For this review, use the dimensioned drawing (mm, ordinates from the lowest corner) and the shaded views. Round coordinates to 2 decimals unless told otherwise and drop trailing zeros. Write each loop counter-clockwise with the first axis right and the second up, starting at its lowest first coordinate (ties: lowest second). Pieces come first, ordered by that corner, then holes.
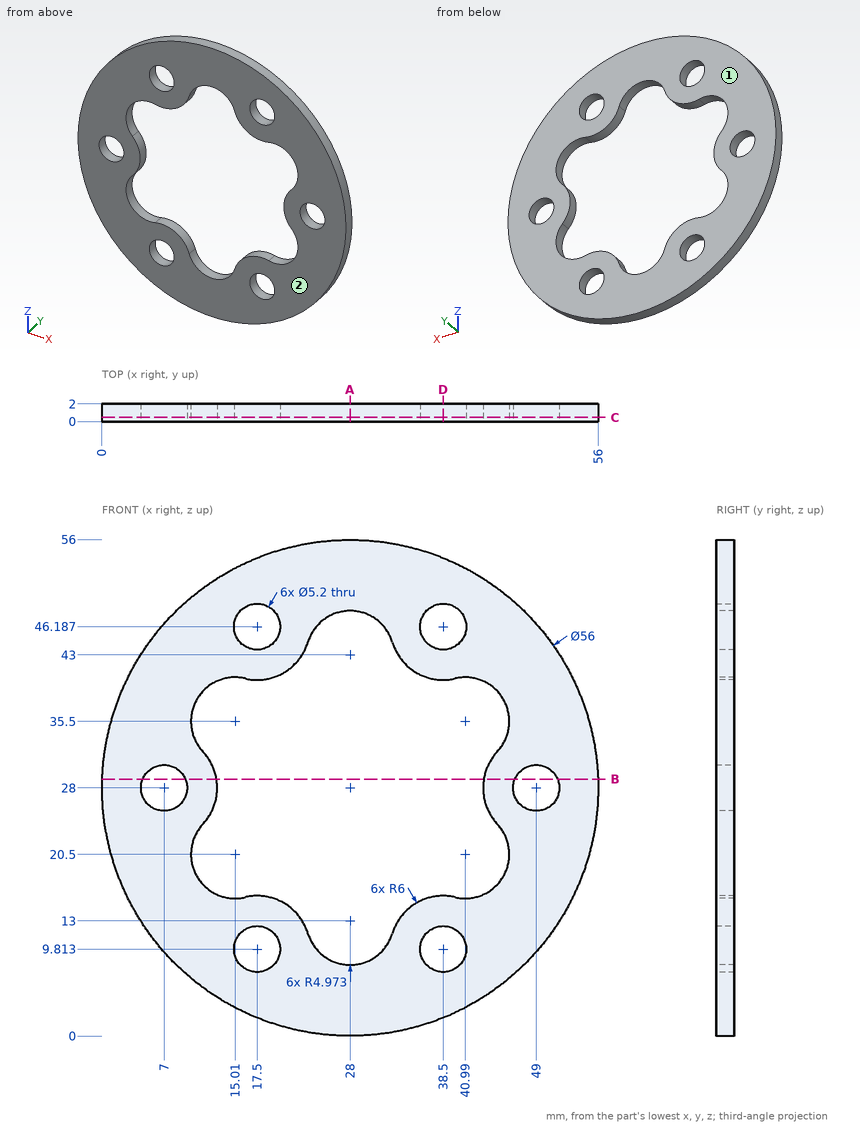
1) Add section A-A on x = 28. State the section outline as (y, z) points, and give its area (3 significant figures).
2) Add section B-B on z = 29. State the section outline as (x, y) points.
3) For line 1 along X through (y, z) = (0.1, 29) (1 decimal); line 2 along Z through (x, y) = (16.5, 0.8) (1 decimal); line 3 along Z through (x, y) = (38, 1) (1 decimal), list the stretches that pass through material, from the lowest coordinate up.
4) Add section D-D on x = 38.5. State the section outline as (y, z) points.
5) The part is to be moulded in two halves that separate along Y. For the marked faces 1 and 2, say which applies: pulls with the +Y half, pulls with the -Y half, needs draft (parallel to the pull), parting line crosses it, or undercut.
6) Add section C-C on y = 0.5. State the section outline as (x, z) points (1 decimal).
7) For P1, Ø7, axis at x = 38.5, z = 46.19, coming from the +Y side; P2, Ø4, axis at x = 17.5, z = 46.19, coming from the -Y side, all flat-tipped, find the tip position at first contact; note any pin that passes through.
Computed:
1. outline: (0, 0) - (2, 0) - (2, 8.03) - (0, 8.03) - close; (0, 47.97) - (2, 47.97) - (2, 56) - (0, 56) - close
1. area: 32.1 mm2
2. outline: (0.02, 0) - (4.6, 0) - (4.6, 2) - (0.02, 2) - close; (9.4, 0) - (12.92, 0) - (12.92, 2) - (9.4, 2) - close; (43.08, 0) - (46.6, 0) - (46.6, 2) - (43.08, 2) - close; (51.4, 0) - (55.98, 0) - (55.98, 2) - (51.4, 2) - close
3. line 1: x = 0 to 4.6, 9.4 to 12.9, 43.1 to 46.6, 51.4 to 56
3. line 2: z = 2.5 to 7.4, 12.2 to 15.7, 40.3 to 43.8, 48.6 to 53.5
3. line 3: z = 1.8 to 7.3, 12.4 to 15.8, 40.2 to 43.6, 48.7 to 54.2
4. outline: (0, 2.04) - (2, 2.04) - (2, 7.21) - (0, 7.21) - close; (0, 12.41) - (2, 12.41) - (2, 15.81) - (0, 15.81) - close; (0, 40.19) - (2, 40.19) - (2, 43.59) - (0, 43.59) - close; (0, 48.79) - (2, 48.79) - (2, 53.96) - (0, 53.96) - close
5. face 1: pulls with the +Y half
5. face 2: pulls with the -Y half
6. outline: circle Ø56 at (28, 28); hole circle Ø5.2 at (7, 28); hole (11.4, 23.9) arc R5 ccw to (16.1, 15.7) arc R6 cw to (23.2, 11.6) arc R5 ccw to (32.8, 11.6) arc R6 cw to (39.9, 15.7) arc R5 ccw to (44.6, 23.9) arc R6 cw to (44.6, 32.1) arc R5 ccw to (39.9, 40.3) arc R6 cw to (32.8, 44.4) arc R5 ccw to (23.2, 44.4) arc R6 cw to (16.1, 40.3) arc R5 ccw to (11.4, 32.1) arc R6 cw to start; hole circle Ø5.2 at (17.5, 9.8); hole circle Ø5.2 at (17.5, 46.2); hole circle Ø5.2 at (38.5, 9.8); hole circle Ø5.2 at (38.5, 46.2); hole circle Ø5.2 at (49, 28)
7. P1: stops at y = 2
7. P2: passes through
